```python
from build123d import *

# Parameters (mm, degrees)
F0_R     = 17.54425
F1_DEPTH = 3
F0_R_2   = 12.54425
F2_DEPTH = 3
F3_DEPTH = 11
F4_R     = 2
F5_W     = 33.528
F5_H     = 33.528
F5_W_2   = 3.41975
F5_H_2   = 31.928
F6_DEPTH = 12.7
F7_R     = 1.8
F8_DEPTH = 37.30925


with BuildPart() as f1:
    # F0 (on Front) → F1 (new body)
    with BuildSketch(Plane.XZ):
        with BuildLine():
            ThreePointArc((20.54425, 0), (14.5269784894, 14.5269784894), (0, 20.54425))
            ThreePointArc((0, 20.54425), (-14.5269785029, 14.5269784759), (-20.54425, -3.82e-08))
            ThreePointArc((-20.54425, -3.82e-08), (-14.5269784759, -14.5269785029), (0, -20.54425))
            ThreePointArc((0, -20.54425), (14.5269784894, -14.5269784894), (20.54425, 0))
        make_face()
        Circle(F0_R, mode=Mode.SUBTRACT)
        with BuildLine():
            Line((20.54425, 20.54425), (0, 20.54425))
            ThreePointArc((0, 20.54425), (14.5269784894, 14.5269784894), (20.54425, 0))
            Line((20.54425, 0), (20.54425, 20.54425))
        make_face()
        with BuildLine():
            Line((20.54425, -20.54425), (20.54425, 0))
            ThreePointArc((20.54425, 0), (14.5269784894, -14.5269784894), (0, -20.54425))
            Line((0, -20.54425), (20.54425, -20.54425))
        make_face()
        with BuildLine():
            Line((0, 20.54425), (-20.54425, 20.54425))
            Line((-20.54425, 20.54425), (-20.54425, -3.82e-08))
            ThreePointArc((-20.54425, -3.82e-08), (-14.5269785029, 14.5269784759), (0, 20.54425))
        make_face()
        with BuildLine():
            ThreePointArc((0, -20.54425), (-14.5269784759, -14.5269785029), (-20.54425, -3.82e-08))
            Line((-20.54425, -3.82e-08), (-20.54425, -20.54425))
            Line((-20.54425, -20.54425), (0, -20.54425))
        make_face()
    extrude(amount=F1_DEPTH)

    # F0 (on Front) → F2 (join)
    with BuildSketch(Plane.XZ):
        Circle(F0_R)
        Circle(F0_R_2, mode=Mode.SUBTRACT)
    extrude(amount=F2_DEPTH)

    # F0 (on Front) → F3 (join)
    with BuildSketch(Plane.XZ):
        with BuildLine():
            ThreePointArc((20.54425, 0), (14.5269784894, 14.5269784894), (0, 20.54425))
            ThreePointArc((0, 20.54425), (-14.5269785029, 14.5269784759), (-20.54425, -3.82e-08))
            ThreePointArc((-20.54425, -3.82e-08), (-14.5269784759, -14.5269785029), (0, -20.54425))
            ThreePointArc((0, -20.54425), (14.5269784894, -14.5269784894), (20.54425, 0))
        make_face()
        Circle(F0_R, mode=Mode.SUBTRACT)
    extrude(amount=F3_DEPTH)

    # F4
    f4_edges = [f1.edges().sort_by_distance(p)[0] for p in [
        (-17.54425, -11, 0),
    ]]
    fillet(f4_edges, radius=F4_R)

    # F5 (on Front) → F6 (join)
    with BuildSketch(Plane.XZ):
        Rectangle(F5_W, F5_H)
        Polygon((12.54425, 15.964), (15.964, 15.964), (15.964, -15.964), (12.54425, -15.964), (-12.54425, -15.964), (-15.964, -15.964), (-15.964, 15.964), (-12.54425, 15.964), align=None, mode=Mode.SUBTRACT)
        with Locations((14.254125, 0)):
            Rectangle(F5_W_2, F5_H_2)
        with Locations((-14.254125, 0)):
            Rectangle(F5_W_2, F5_H_2)
    extrude(amount=-F6_DEPTH)

    # F7 (on face) → F8 (cut, through all)
    with BuildSketch(Plane.YZ.offset(16.764)):
        with Locations((5.5796158184, 13.4703841816)):
            Circle(F7_R)
        with Locations((5.5796158184, -13.4703841816)):
            Circle(F7_R)
    extrude(amount=-F8_DEPTH, mode=Mode.SUBTRACT)


solid = f1.part
```
Input: part model. Units: mm. Frame: model coordinates. A direction names the side the tool comes from. Coordinates: 2 decimals unless noted, no trailing zeros. Loops run counter-clockwise (first coordinate to the right, second up) from the corner with the lowest first, then second, coordinate; pieces in that order, holes last. Notation, with made-up numbers: (47.25, 43) -> (55.25, 43) arc R17 cw to (55.25, 48) -> close; hole circle Ø8 at (-38.5, 24). An arc over 180 degrees is marked (long way). Use a Markdown table: item, result.
1) Access query for faces 4 (the flat face through (8, -3, -11)), 5 (the flat face through (16, -3, 16)), 6 (the flat face through (-16, -3, -16)), 7 (the flat face through (0, 6, 15.964)). Directions: +Z, -Z, +X, -X, +Y, -Y. A direction counts if a zero-diameter tool reaches every point of the face in a straight line with its end or side. Return the directions, or none.
Results found:
| item | result |
|---|---|
| face 4 | -Y |
| face 5 | +Z, +X, -Y |
| face 6 | -Z, -X, -Y |
| face 7 | +Y |
2) Material intervals for line 1 along X through (y, z) = (5.25, -6); line 2 along Z through (x, y) = (6, 1.5); line 3 along Y through (x, z) = (10, 19), sorted ascending. Write a range as from..to.
Results found:
| item | result |
|---|---|
| line 1 | x = -16.76..-12.54, 12.54..16.76 |
| line 2 | z = -16.76..-15.96, 15.96..16.76 |
| line 3 | y = -3..0 |
3) Cut plane C-C (y = -4.75). Return the cut outline in (x, z), then the cut area to 3 significant figures.
Results found:
| item | result |
|---|---|
| outline | circle Ø41.09 at (0, 0); hole circle Ø35.09 at (0, 0) |
| area | 359 mm2 |
4) Contact query for flat-ended pins moving along their axis: pin 1 (4 mm diameter, centred on y = 8.5, z = -1, fed in from -X); pin 2 (12 mm diameter, centred on x = -5.5, y = 7, fed in from +Z); pin 3 (12 mm diameter, centred on x = -0.5, z = -7, fed in from -Y). Output: stop coordinate, or through.
Results found:
| item | result |
|---|---|
| pin 1 | stops at x = -16.76 |
| pin 2 | stops at z = 16.76 |
| pin 3 | stops at y = -3 |
5) Cut plane A-A (y = 10.5). Return the cut outline in (x, z), then the cut area to 3 significant figures.
Results found:
| item | result |
|---|---|
| outline | (-16.76, -16.76) -> (16.76, -16.76) -> (16.76, 16.76) -> (-16.76, 16.76) -> close; hole (-12.54, -15.96) -> (12.54, -15.96) -> (12.54, 15.96) -> (-12.54, 15.96) -> close |
| area | 323 mm2 |
6) Pull-direction query (X, two-part tool) for faces 1 (the flat face through (-20.544, -1, 0)), 2 (the flat face through (0, 0, -13)), 3 (the cylindrical face through (14.684, 6.41, 11.873)); classes: released by +X, released by -X, zero draft, split by the parting line, or undercut.
Results found:
| item | result |
|---|---|
| face 1 | released by -X |
| face 2 | undercut |
| face 3 | zero draft |
7) Cut plane B-B (x = -14.5). Give the number of separate pieces and of enclosed holes in the cut face, then the cut area to 3 significant figures.
Results found:
| item | result |
|---|---|
| separate pieces | 1 |
| enclosed holes | 2 |
| area | 601 mm2 |
